```python
from build123d import *

# Parameters (mm, degrees)
EXTRUDE_1_DEPTH = 4
EXTRUDE_3_DEPTH = 100


with BuildPart() as part:
    # 草图1 → 凸台-拉伸1 (new body)
    with BuildSketch(Plane(origin=(0, 0, 0), x_dir=(1, 0, 0), z_dir=(0, 1, 0))):
        with BuildLine():
            ThreePointArc((50, 45), (48.535533906, 48.535533906), (45, 50))
            Line((45, 50), (-29.154564109, 50))
            Line((-29.154564109, 50), (-29.151954818, 49.997335451))
            Line((-29.151954818, 49.997335451), (-29.408928245, 49.745691122))
            Line((-29.408928245, 49.745691122), (-29.657963283, 50))
            Line((-29.657963283, 50), (-45, 50))
            ThreePointArc((-45, 50), (-48.535533906, 48.535533906), (-50, 45))
            Line((-50, 45), (-50, -45))
            ThreePointArc((-50, -45), (-48.535533906, -48.535533906), (-45, -50))
            Line((-45, -50), (45, -50))
            ThreePointArc((45, -50), (48.535533906, -48.535533906), (50, -45))
            Line((50, -45), (50, 45))
        make_face()
    extrude(amount=EXTRUDE_1_DEPTH)

    # 草图2 → 凸台-拉伸3 (add)
    with BuildSketch(Plane(origin=(0, 4, 0), x_dir=(1, 0, 0), z_dir=(0, 1, 0))):
        with BuildLine():
            Line((45, 50), (-45, 50))
            ThreePointArc((-45, 50), (-48.535533906, 48.535533906), (-50, 45))
            Line((-50, 45), (-50, -45))
            ThreePointArc((-50, -45), (-48.535533906, -48.535533906), (-45, -50))
            Line((-45, -50), (45, -50))
            ThreePointArc((45, -50), (48.535533906, -48.535533906), (50, -45))
            Line((50, -45), (50, 45))
            ThreePointArc((50, 45), (48.535533906, 48.535533906), (45, 50))
        make_face()
        with BuildLine():
            Line((-47, 45), (-47, -40.171572875))
            ThreePointArc((-47, -40.171572875), (-45.765366865, -42.01933194), (-43.585786438, -41.585786438))
            Line((-43.585786438, -41.585786438), (41.585786438, 43.585786438))
            ThreePointArc((41.585786438, 43.585786438), (42.01933194, 45.765366865), (40.171572875, 47))
            Line((40.171572875, 47), (-45, 47))
            ThreePointArc((-45, 47), (-46.414213562, 46.414213562), (-47, 45))
        make_face(mode=Mode.SUBTRACT)
        with BuildLine():
            Line((-40.171572875, -47), (45, -47))
            ThreePointArc((45, -47), (46.414213562, -46.414213562), (47, -45))
            Line((47, -45), (47, 40.171572875))
            ThreePointArc((47, 40.171572875), (45.765366865, 42.01933194), (43.585786438, 41.585786438))
            Line((43.585786438, 41.585786438), (-41.585786438, -43.585786438))
            ThreePointArc((-41.585786438, -43.585786438), (-42.01933194, -45.765366865), (-40.171572875, -47))
        make_face(mode=Mode.SUBTRACT)
    extrude(amount=EXTRUDE_3_DEPTH)


solid = part.part
```
CAD build for the part. Positions are in the model's coordinates, mm. A direction names the side the tool comes from. Round coordinates to 2 decimals unless told otherwise and drop trailing zeros. Write each loop counter-clockwise with the first axis right and the second up, starting at its lowest first coordinate (ties: lowest second). Pieces come first, ordered by that corner, then holes. Notation, with made-up numbers: (52.5, 80.5) - (83.5, 80.5) arc R21 cw to (83.5, 90.5) - close; hole circle Ø11 at (58.25, -32). An arc over 180 degrees is marked (long way). Return JSON: item names as keys, results as strings. Group by question number.
Item 1: Mould opens along X. For faces 1 (the face through (-50, 51, -1)), 2 (the face through (1, 51, -50)), 3 (the face through (2, 53, 47)), 4 (the face through (48, 51, 49)) say: +X half, -X half, draft (parallel to the pull), parting line (faces both ways), or undercut.
Item 2: 3-axis set-ups, long thin cutter, end or side, ignore diameter. For faces 5 (the face through (-47, 53, -3)), 6 (the face through (50, 51, 1)): which of +Z, -Z, +X, -X, +Y, -Y reach the whole face in a straight line?
Item 3: Probe probe 1 along X at (y, z) = (99.5, 16.5); probe 2 along X at (y, z) = (24, -5.5); probe 3 along Z at (x, y) = (9.5, 21). List the from-to ranges inside material, lowest first.
Item 4: Flat gauge pin, fed straight in: pin 1 Ø8 at (x, z) = (-1.5, 24) entering from +Y. Where does the tip first touch, or does it go through?
Item 5: Band-saw the part on C-C on x = 22. List the corners of the cut face in (y, z).
Item 6: Band-saw the part on B-B on z = -12.5. List the corners of the cut face in (x, y), plus the area to 3 significant figures.
Item 7: Band-saw the part on A-A on y = 11.5. List the corners of the cut face in (x, z).
Resolved:
{
 "1": {"face 1": "-X half", "face 2": "draft", "face 3": "undercut", "face 4": "+X half"},
 "2": {"face 5": "+Y", "face 6": "+Z, -Z, +X, +Y, -Y"},
 "3": {"probe 1": "x = -50 to -47, -18.5 to -14.5, 47 to 50", "probe 2": "x = -50 to -47, 3.5 to 7.5, 47 to 50", "probe 3": "z = -50 to -47, -11.5 to -7.5, 47 to 50"},
 "4": {"pin 1": "stops at y = 4"},
 "5": {"outline": "(0, -50) - (104, -50) - (104, -47) - (4, -47) - (4, -24) - (104, -24) - (104, -20) - (4, -20) - (4, 47) - (104, 47) - (104, 50) - (0, 50) - close"},
 "6": {"outline": "(-50, 0) - (50, 0) - (50, 104) - (47, 104) - (47, 4) - (14.5, 4) - (14.5, 104) - (10.5, 104) - (10.5, 4) - (-47, 4) - (-47, 104) - (-50, 104) - close", "area": "1,400 mm²"},
 "7": {"outline": "(-50, -45) arc R5 ccw to (-45, -50) - (45, -50) arc R5 ccw to (50, -45) - (50, 45) arc R5 ccw to (45, 50) - (-45, 50) arc R5 ccw to (-50, 45) - close; hole (-47, -45) arc R2 ccw to (-45, -47) - (40.17, -47) arc R2 ccw to (41.59, -43.59) - (-43.59, 41.59) arc R2 ccw to (-47, 40.17) - close; hole (-41.59, 43.59) - (43.59, -41.59) arc R2 ccw to (47, -40.17) - (47, 45) arc R2 ccw to (45, 47) - (-40.17, 47) arc R2 ccw to start"}
}
